Answer from the drawing. Dimensions are ordinates in mm from the lowest x, y and z of the part. Round coordinates to 2 decimals unless told otherwise and drop trailing zeros. Loops run counter-clockwise (first coordinate to the right, second up) from the corner with the lowest first, then second, coordinate; pieces in that order, holes last. Notation, with made-up numbers: (-39.5, 57.25) - (-11.5, 57.25) arc R25 cw to (-11.5, 82.25) - close; hole circle Ø9 at (26.5, -4.75). An arc over 180 degrees is marked (long way). Write item = value, one per line. Start each with the question number.
1) For a pull along Z with two mould halves and no side action, classify the marked faces 1, 2 and 3 as released by +Z, released by -Z, zero draft, split by the parting line, or undercut.
2) Section D-D, the plane z = 20 is taken. Determine the outline of the cut face in (x, y).
3) Section B-B, the plane y = 35 is taken. Determine the outline of the cut face in (x, z).
4) Section C-C, the plane x = 25 is taken. Determine the outline of the cut face in (y, z).
5) Straight lines are drawn through the part: line 1 along Z through (x, y) = (25, 2); line 2 along Z through (x, y) = (48.9, 20); line 3 along X through (y, z) = (11.5, 34.5). For each, find the intervals that lie inside material, in ascending order.
6) Given pin 1 Ø9 at (x, z) = (25, 20) entering from -Y; pin 2 Ø6 at (x, z) = (29, 27) entering from +Y; pin 3 Ø1 at (x, y) = (26.5, 7) entering from +Z; pin 4 Ø12 at (x, z) = (35, 26) entering from +Y, each flat-ended and moving along its own axis, determine where each tip first touches the part or whether it passes through.
7) Section A-A, the plane z = 30 is taken. Determine the outline of the cut face in (x, y), and give its area (3 significant figures).
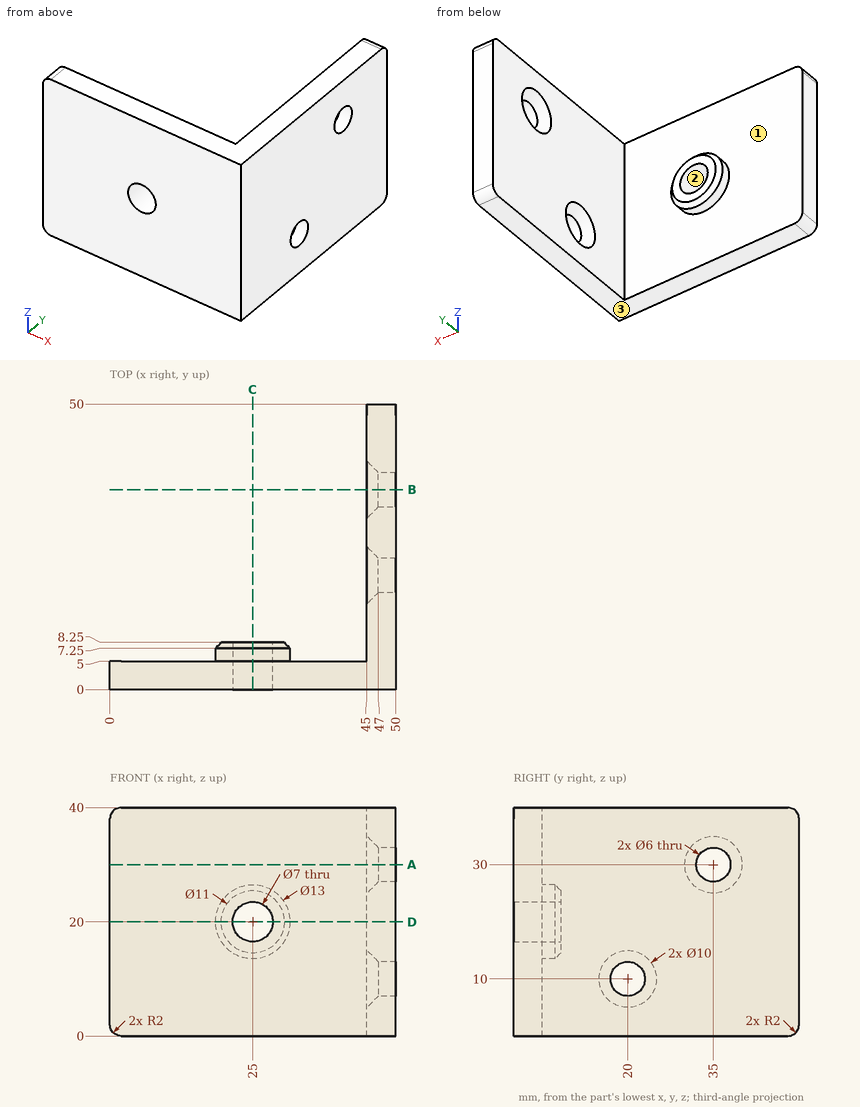
Geometry check:
q1.face_1 = zero draft
q1.face_2 = undercut
q1.face_3 = released by -Z
q2.outline = (0, 0) - (21.5, 0) - (21.5, 8.25) - (19.5, 8.25) - (18.5, 7.25) - (18.5, 5) - (0, 5) - close; (28.5, 0) - (50, 0) - (50, 50) - (45, 50) - (45, 5) - (31.5, 5) - (31.5, 7.25) - (30.5, 8.25) - (28.5, 8.25) - close
q3.outline = (45, 0) - (50, 0) - (50, 27) - (47, 27) - (45, 25) - close; (45, 35) - (47, 33) - (50, 33) - (50, 40) - (45, 40) - close
q4.outline = (0, 0) - (5, 0) - (5, 13.5) - (7.25, 13.5) - (8.25, 14.5) - (8.25, 16.5) - (0, 16.5) - close; (0, 23.5) - (8.25, 23.5) - (8.25, 25.5) - (7.25, 26.5) - (5, 26.5) - (5, 40) - (0, 40) - close
q5.line_1 = 0 to 16.5, 23.5 to 40
q5.line_2 = 0 to 7, 13 to 40
q5.line_3 = 45 to 50
q6.pin_1 = 0
q6.pin_2 = 8.25
q6.pin_3 = 26.42
q6.pin_4 = 8.09
q7.outline = (0, 0) - (50, 0) - (50, 32) - (47, 32) - (45, 30) - (45, 5) - (0, 5) - close; (45, 40) - (47, 38) - (50, 38) - (50, 50) - (45, 50) - close
q7.area = 441 mm2
